from build123d import *

# Parameters (mm, degrees)
F3_DEPTH        = 5.08
F4_R            = 6.35
F5_SIZE         = 3.048
F7_DEPTH        = 12.7
F7_COPIES_COUNT = 3


# Not quite as in the source:
# - a pattern or mirror of a feature is missing from the dataset's text; its kind, count and spacing are read off the source's solid


with BuildPart() as f3:
    # F2 (on Top) → F3 (new body, symmetric)
    with BuildSketch(Plane.XY):
        Polygon((7.1554966211, 22.3350380043), (5.08, 38.1), (-5.08, 38.1), (-7.1554966211, 22.3350380043), (-13.2405448196, 7.6444321158), (-22.9204586168, -4.9706771516), (-35.5355678842, -14.6505909488), (-30.4555678842, -23.4494090512), (-15.7649619957, -17.3643608527), (0, -15.2888642316), (15.7649619957, -17.3643608527), (30.4555678842, -23.4494090512), (35.5355678842, -14.6505909488), (22.9204586168, -4.9706771516), (13.2405448196, 7.6444321158), align=None)
    extrude(amount=F3_DEPTH, both=True)

    # F4
    f4_edges = [f3.edges().sort_by_distance(p)[0] for p in [
        (-22.920459, -4.970677, 0),
        (-13.240545, 7.644432, 0),
        (7.155497, 22.335038, 0),
        (13.240545, 7.644432, 0),
        (-15.764962, -17.364361, 0),
        (0, -15.288864, 0),
        (22.920459, -4.970677, 0),
        (-7.155497, 22.335038, 0),
        (15.764962, -17.364361, 0),
    ]]
    fillet(f4_edges, radius=F4_R)

    # F5
    f5_edges = [f3.edges().sort_by_distance(p)[0] for p in [
        (-23.496444, -20.566845, 5.08),
        (-7.882481, -16.326613, 5.08),
        (7.882481, -16.326613, 5.08),
        (-29.559632, -10.065094, 5.08),
        (-18.080502, 1.336877, 5.08),
        (-10.198021, 14.989735, 5.08),
        (6.063189, 30.63194, 5.08),
        (10.198021, 14.989735, 5.08),
        (18.080502, 1.336877, 5.08),
        (-29.559632, -10.065094, -5.08),
        (-18.080502, 1.336877, -5.08),
        (-10.198021, 14.989735, -5.08),
        (6.063189, 30.63194, -5.08),
        (10.198021, 14.989735, -5.08),
        (18.080502, 1.336877, -5.08),
        (7.882481, -16.326613, -5.08),
        (-7.882481, -16.326613, -5.08),
        (-23.496444, -20.566845, -5.08),
        (-15.75078, -17.417288, -5.08),
        (0, -15.343658, -5.08),
        (15.75078, -17.417288, -5.08),
        (23.496444, -20.566845, -5.08),
        (-22.959204, -4.931932, -5.08),
        (29.559632, -10.065094, -5.08),
        (-13.287998, 7.671829, -5.08),
        (22.959204, -4.931932, -5.08),
        (-7.208423, 22.34922, -5.08),
        (13.287998, 7.671829, -5.08),
        (-6.063189, 30.63194, -5.08),
        (7.208423, 22.34922, -5.08),
        (-15.75078, -17.417288, 5.08),
        (0, -15.343658, 5.08),
        (15.75078, -17.417288, 5.08),
        (23.496444, -20.566845, 5.08),
        (-22.959204, -4.931932, 5.08),
        (29.559632, -10.065094, 5.08),
        (-13.287998, 7.671829, 5.08),
        (22.959204, -4.931932, 5.08),
        (-7.208423, 22.34922, 5.08),
        (13.287998, 7.671829, 5.08),
        (-6.063189, 30.63194, 5.08),
        (7.208423, 22.34922, 5.08),
    ]]
    chamfer(f5_edges, length=F5_SIZE)

    # F6 (on face) → F7 (cut)
    with BuildSketch(Plane(origin=(32.9955678842, -19.05, 0), x_dir=(0.5, 0.8660254038, 0), z_dir=(0.8660254038, -0.5, 0))):
        Polygon((-1.8330871047, 3.175), (-3.6661742094, 0), (-1.8330871047, -3.175), (1.8330871047, -3.175), (3.6661742094, 0), (1.8330871047, 3.175), align=None)
    f7 = extrude(amount=-F7_DEPTH, mode=Mode.SUBTRACT)

    # F7_copies: F7 ×3 about axis
    f7_copies_axis = Axis((0, 0, 0), (0, 0, 1))
    for i in range(1, F7_COPIES_COUNT):
        add(f7.rotate(f7_copies_axis, i * 360 / F7_COPIES_COUNT), mode=Mode.SUBTRACT)


solid = f3.part
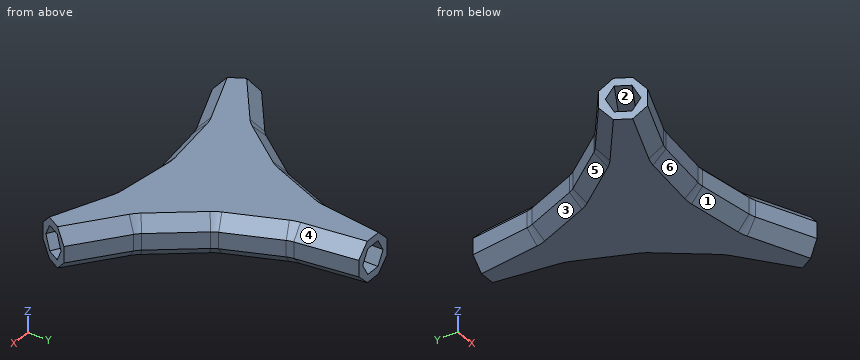
Verification items for the finished model (mm, model axes). Face numbers are marked on the shaded views. A direction names the side the tool comes from. Round coordinates to 2 decimals unless told otherwise and drop trailing zeros. Write each loop counter-clockwise with the first axis right and the second up, starting at its lowest first coordinate (ties: lowest second). Pieces come first, ordered by that corner, then holes.
(1) Section check B-B (y = 13.5). Enter the section's corners in (x, z).
Returned:
outline: (-10.82, -2.03) - (-7.52, -5.08) - (7.52, -5.08) - (10.82, -2.03) - (10.82, 2.03) - (7.52, 5.08) - (-7.52, 5.08) - (-10.82, 2.03) - close
(2) Access from +Z, -Z, +X, -X, +Y, -Y to the whole of each face (thin tool, end or side, straight path). Record for the marked faces 1, 2 and 3.
Returned:
face 1: -Z, -Y
face 2: none
face 3: -Z, -X, +Y
(3) Mould release check, pull along X, two halves, no side actions. Record for the marked faces 4, 5 and 6: pulls with the +X half, pulls with the -X half, needs draft (parallel to the pull), parting line crosses it, or undercut.
Returned:
face 4: pulls with the +X half
face 5: pulls with the -X half
face 6: undercut
(4) Section check C-C (z = -4). Enter the section's corners in (x, y).
Returned:
outline: (-34.54, -16.37) - (-31.45, -21.73) - (-17.29, -15.87) arc R8.32 cw to (-15.19, -15.3) - (-1.09, -13.45) arc R8.32 cw to (1.09, -13.45) - (15.19, -15.3) arc R8.32 cw to (17.29, -15.87) - (31.45, -21.73) - (34.54, -16.37) - (22.39, -7.04) arc R8.32 cw to (20.85, -5.51) - (12.19, 5.78) arc R8.32 cw to (11.1, 7.66) - (5.66, 20.81) arc R8.32 cw to (5.1, 22.91) - (3.1, 38.1) - (-3.1, 38.1) - (-5.1, 22.91) arc R8.32 cw to (-5.66, 20.81) - (-11.1, 7.66) arc R8.32 cw to (-12.19, 5.78) - (-20.85, -5.51) arc R8.32 cw to (-22.39, -7.04) - close
(5) Section check D-D (x = -19). Enter the section's corners in (y, z).
Returned:
outline: (-18.7, -2.03) - (-15.41, -5.08) - (-4.87, -5.08) - (0.14, -2.03) - (0.14, 2.03) - (-4.87, 5.08) - (-15.41, 5.08) - (-18.7, 2.03) - close
(6) Depth check by flat-ended pin: pin 1 Ø6 at (x, z) = (15.5, -1) entering from -Y; pin 2 Ø1.9 at (x, z) = (1.5, 1) entering from +Y; pin 3 Ø1 at (x, z) = (-22, 3.5) entering from -Y; pin 4 Ø12 at (x, y) = (17.5, -16) entering from +Z. Enter the tip coordinate at first touch or a pass-through.
Returned:
pin 1: stops at y = -18.5
pin 2: stops at y = 25.4
pin 3: stops at y = -18.94
pin 4: stops at z = 5.08
(7) Section check A-A (x = 26). Enter the section's corners in (y, z) (3 decimals), plus the area to 3 significant figures.
Returned:
outline: (-21.604, -2.032) - (-18.305, -5.08) - (-11.176, -5.08) - (-7.334, -2.032) - (-7.334, 2.032) - (-11.176, 5.08) - (-18.305, 5.08) - (-21.604, 2.032) - close; hole (-19.244, 0) - (-17.128, -3.175) - (-12.894, -3.175) - (-10.778, 0) - (-12.894, 3.175) - (-17.128, 3.175) - close
area: 82.9 mm2
(8) Material ranges on line 1 (Z direction, x = 0.5, y = 26.5) (3 decimals); line 2 (X direction, y = -13, z = 0.75); line 3 (Y direction, x = -20.5, z = -0.75), recorded low to high.
Returned:
line 1: z = -5.08 to -3.175, 3.175 to 5.08
line 2: x = -33.38 to -28.98, -21.82 to 21.82, 28.98 to 33.38
line 3: y = -19.33 to -15.57, -15.29 to -1.82
